Could you check a few things on this model? Use its own coordinates, in mm. A direction names the side the tool comes from. Give positions to 0.01 mm unless a question says otherwise; leave off trailing zeros. Write each loop counter-clockwise with the first axis right and the second up, starting at its lowest first coordinate (ties: lowest second). Pieces come first, ordered by that corner, then holes. Notation, with made-up numbers: (-35, -24) -> (15, -24) arc R25 cw to (15, 8) -> close; hole circle Ø4 at (48, -36). An arc over 180 degrees is marked (long way). Write item = value, one per line. Start each with the question number.
```python
from build123d import *

# Parameters (mm, degrees)
EXTRUDE_1_DEPTH           = 6
FILLET_1_R                = 1
EXTRUDE_2_DEPTH           = 3
FILLET_2_R                = 2
HOLE_WIZARD_1_D           = 3.4
HOLE_WIZARD_1_CBORE_D     = 5
HOLE_WIZARD_1_CBORE_DEPTH = 3.4
EXTRUDE_3_DEPTH           = 1
CHAMFER_1_SIZE            = 0.5


with BuildPart() as part:
    # 草图1 → 凸台-拉伸1 (new body)
    with BuildSketch(Plane.XY):
        with BuildLine():
            Line((-5.26394944, 46.201091289), (-5.943168723, 52.162522423))
            ThreePointArc((-5.943168723, 52.162522423), (0, 52.5), (5.943168723, 52.162522423))
            Line((5.943168723, 52.162522423), (5.26394944, 46.201091289))
            ThreePointArc((5.26394944, 46.201091289), (0, 46.5), (-5.26394944, 46.201091289))
        make_face()
    extrude(amount=EXTRUDE_1_DEPTH)

    # 圆角1
    fillet_1_edges = [part.edges().sort_by_distance(p)[0] for p in [
        (5.943168723, 52.162522423, 3),
        (5.26394944, 46.201091289, 3),
        (-5.26394944, 46.201091289, 3),
        (-5.943168723, 52.162522423, 3),
    ]]
    fillet(fillet_1_edges, radius=FILLET_1_R)

    # 草图2 → 凸台-拉伸2 (add)
    with BuildSketch(Plane.XY.offset(6)):
        with BuildLine():
            Line((-9.198683592, 41.492580303), (-11.363079732, 51.255540374))
            ThreePointArc((-11.363079732, 51.255540374), (0, 52.5), (11.363079732, 51.255540374))
            Line((11.363079732, 51.255540374), (9.198683592, 41.492580303))
            ThreePointArc((9.198683592, 41.492580303), (0, 42.5), (-9.198683592, 41.492580303))
        make_face()
    extrude(amount=EXTRUDE_2_DEPTH)

    # 圆角2
    fillet_2_edges = [part.edges().sort_by_distance(p)[0] for p in [
        (11.363079732, 51.255540374, 7.5),
        (-11.363079732, 51.255540374, 7.5),
        (-9.198683592, 41.492580303, 7.5),
        (9.198683592, 41.492580303, 7.5),
    ]]
    fillet(fillet_2_edges, radius=FILLET_2_R)

    # 打孔尺寸(%根据)内六角圆柱头螺钉的类型1 (through all)
    with Locations(Plane.XY.offset(9)):
        with Locations((0, 49.5)):
            CounterBoreHole(HOLE_WIZARD_1_D / 2, HOLE_WIZARD_1_CBORE_D / 2, HOLE_WIZARD_1_CBORE_DEPTH)

    # 草图6 → 凸台-拉伸3 (add)
    with BuildSketch(Plane(origin=(0, 0, 6), x_dir=(-1, 0, 0), z_dir=(0, 0, -1))):
        with BuildLine():
            Line((-6.822438201, 51.046100115), (-6.369532765, 47.071000121))
            ThreePointArc((-6.369532765, 47.071000121), (-5.643826215, 45.74538326), (-4.197867409, 45.305936799))
            ThreePointArc((-4.197867409, 45.305936799), (0, 45.5), (4.197867409, 45.305936799))
            ThreePointArc((4.197867409, 45.305936799), (5.643826215, 45.74538326), (6.369532765, 47.071000121))
            Line((6.369532765, 47.071000121), (6.822438201, 51.046100115))
            ThreePointArc((6.822438201, 51.046100115), (6.812927902, 51.570778372), (6.667268559, 52.074922275))
            ThreePointArc((6.667268559, 52.074922275), (5.799030491, 52.178743233), (4.929183703, 52.268089194))
            ThreePointArc((4.929183703, 52.268089194), (5.611821641, 51.902590333), (5.828866345, 51.159303329))
            Line((5.828866345, 51.159303329), (5.375960909, 47.184203334))
            ThreePointArc((5.375960909, 47.184203334), (5.013107634, 46.521394904), (4.290128231, 46.301671673))
            ThreePointArc((4.290128231, 46.301671673), (0, 46.5), (-4.290128231, 46.301671673))
            ThreePointArc((-4.290128231, 46.301671673), (-5.013107634, 46.521394904), (-5.375960909, 47.184203334))
            Line((-5.375960909, 47.184203334), (-5.828866345, 51.159303329))
            ThreePointArc((-5.828866345, 51.159303329), (-5.611821641, 51.902590333), (-4.929183703, 52.268089194))
            ThreePointArc((-4.929183703, 52.268089194), (-5.799030491, 52.178743233), (-6.667268559, 52.074922275))
            ThreePointArc((-6.667268559, 52.074922275), (-6.812927902, 51.570778372), (-6.822438201, 51.046100115))
        make_face()
    extrude(amount=EXTRUDE_3_DEPTH)

    # 倒角1
    chamfer_1_edges = [part.edges().sort_by_distance(p)[0] for p in [
        (0, 46.5, 0),
        (0, 52.5, 0),
        (5.602413627, 49.171753332, 0),
        (-5.602413627, 49.171753332, 0),
        (-5.611821641, 51.902590333, 0),
        (5.611821641, 51.902590333, 0),
        (5.013107634, 46.521394904, 0),
        (-5.013107634, 46.521394904, 0),
    ]]
    chamfer(chamfer_1_edges, length=CHAMFER_1_SIZE)


solid = part.part
```
(1) On a 3-axis mill with a long thin cutter (end or side, diameter ignored), from which of +Z, -Z, +X, -X, +Y, -Y can I reach the whole of each face in a straight line? I mean faces 5 (the flat face through (6.6, 49.1, 5.5)), 6 (the flat face through (-6.593, 49.031, 5.507)), 7 (the cylindrical face through (0.1, 45.5, 5.5)), 8 (the cylindrical face through (-6.814, 51.563, 5.507)). Say none if no direction works.
(2) Imagine slicing it at B-B (z = 1). Please give me the cut outline in (x, y), then the cut area to 3 significant figures.
(3) We'd pull the mould along X, two halves only. Please class faces 1 (the cylindrical face through (6.81, 51.58, 5.51)), 2 (the cylindrical face through (0.1, 46.5, 2.7)), 3 (the flat face through (0, 46, 9)), 4 (the flat face through (2, 49, 5.6)): released by +X, released by -X, zero draft, split by the parting line, or undercut.
(4) Imagine slicing it at D-D (z = 7.75). Please give me the cut outline in (x, y), then the cut area to 3 significant figures.
(5) Imagine slicing it at A-A (x = 0). Please give me the cut outline in (y, z), then the cut area to 3 significant figures.
(6) If I drill on line 1 along Y through (x, z) = (0, 7.7); line 2 along Y through (x, z) = (0, 2.1); line 3 along Z through (x, y) = (-1.5, 48), over which ranges is the centre line in solid material (lowest first)? Write a range as from..to.
(7) I'm going to push flat-ended pins straight in: pin 1 (4 mm diameter, centred on x = 0, y = 49.5, fed in from +Z); pin 2 (2 mm diameter, centred on x = 4.5, z = 7.5, fed in from -Y). Where does each tip first touch, or does it pass through?
(8) Imagine slicing it at C-C (y = 49.5). Please give me the cut outline in (x, z).
Answers below:
q1.face_5 = -Z, +X, -Y
q1.face_6 = -Z, -X, -Y
q1.face_7 = -Z, -Y
q1.face_8 = -Z, -X
q2.outline = (-5.83, 51.16) -> (-5.38, 47.18) arc R1 ccw to (-4.29, 46.3) arc R46.5 cw to (4.29, 46.3) arc R1 ccw to (5.38, 47.18) -> (5.83, 51.16) arc R1 ccw to (4.93, 52.27) arc R52.5 ccw to (-4.93, 52.27) arc R1 ccw to start; hole circle Ø3.4 at (0, 49.5)
q2.area = 57.5 mm^2
q3.face_1 = released by +X
q3.face_2 = undercut
q3.face_3 = zero draft
q3.face_4 = undercut
q4.outline = (-10.92, 49.26) -> (-9.62, 43.4) arc R2 ccw to (-7.32, 41.86) arc R42.5 cw to (7.32, 41.86) arc R2 ccw to (9.62, 43.4) -> (10.92, 49.26) arc R2 ccw to (9.32, 51.67) arc R52.5 ccw to (-9.32, 51.67) arc R2 ccw to start; hole circle Ø5 at (0, 49.5)
q4.area = 184 mm^2
q5.outline = (42.5, 6) -> (45.5, 6) -> (45.5, 5) -> (46.5, 5) -> (46.5, 0.5) -> (47, 0) -> (47.8, 0) -> (47.8, 5.6) -> (47, 5.6) -> (47, 9) -> (42.5, 9) -> close; (51.2, 0) -> (52, 0) -> (52.5, 0.5) -> (52.5, 9) -> (52, 9) -> (52, 5.6) -> (51.2, 5.6) -> close
q5.area = 30.7 mm^2
q6.line_1 = 42.5..47, 52..52.5
q6.line_2 = 46.5..47.8, 51.2..52.5
q6.line_3 = 0..5.6
q7.pin_1 = 5.6
q7.pin_2 = 42.14
q8.outline = (-10.96, 6) -> (-6.65, 6) -> (-6.65, 5) -> (-5.64, 5) -> (-5.64, 0.5) -> (-5.14, 0) -> (-1.7, 0) -> (-1.7, 5.6) -> (-2.5, 5.6) -> (-2.5, 9) -> (-10.96, 9) -> close; (1.7, 0) -> (5.14, 0) -> (5.64, 0.5) -> (5.64, 5) -> (6.65, 5) -> (6.65, 6) -> (10.96, 6) -> (10.96, 9) -> (2.5, 9) -> (2.5, 5.6) -> (1.7, 5.6) -> close
